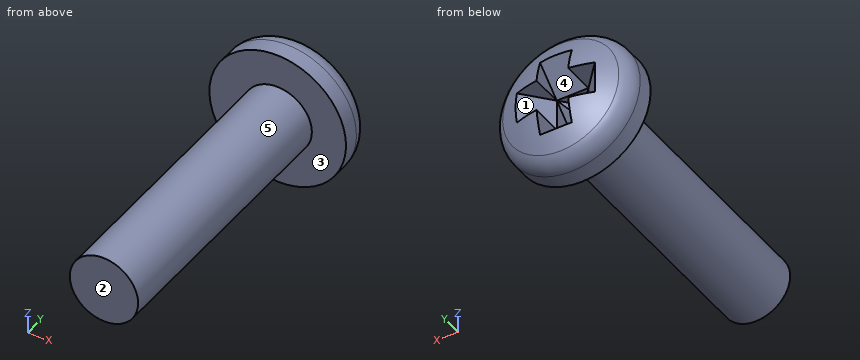
```python
from build123d import *

# Parameters (mm, degrees)
SKETCH2_W          = 1.5875
SKETCH2_H          = 12.7
CUT_EXTRUDE1_DEPTH = 0.736599362
CUT_EXTRUDE2_DEPTH = 0.736599362


with BuildPart() as part:
    # Sketch1 → Base-Revolve (revolve)
    with BuildSketch(Plane.XY, mode=Mode.PRIVATE) as base_revolve_sk:
        with BuildLine():
            Line((0, 0), (3.175, 0))
            Line((3.175, 0), (3.175, 0.762))
            ThreePointArc((3.175, 0.762), (3.047218091, 1.234139911), (2.698756382, 1.577387268))
            ThreePointArc((2.698756382, 1.577387268), (1.395118097, 2.105894374), (0, 2.286))
            Line((0, 2.286), (0, 0))
        make_face()
    revolve(base_revolve_sk.sketch.rotate(Axis((0, 0, 0), (0, 1, 0)), 90), axis=Axis((0, 0, 0), (0, 1, 0)))

    # Sketch2 → Boss-Revolve1 (revolve)
    with BuildSketch(Plane.XY):
        with Locations((0.79375, -6.35)):
            Rectangle(SKETCH2_W, SKETCH2_H)
    revolve(axis=Axis((0, 0, 0), (0, 1, 0)))

    # Sketch3 → Cut-Extrude1 (cut, symmetric)
    with BuildSketch(Plane.XY):
        Polygon((-4.038596502, 6.667494225), (4.038596502, 6.667494225), (4.038596502, 4.44499615), (0, -0.12699989), (-4.038596502, 4.44499615), align=None)
    extrude(amount=CUT_EXTRUDE1_DEPTH, both=True, mode=Mode.SUBTRACT)

    # Sketch4 → Cut-Extrude2 (cut, symmetric)
    with BuildSketch(Plane(origin=(0, 0, 0), x_dir=(0, 0, -1), z_dir=(1, 0, 0))):
        Polygon((-4.038596502, 6.667494225), (4.038596502, 6.667494225), (4.038596502, 4.44499615), (0, -0.12699989), (-4.038596502, 4.44499615), align=None)
    extrude(amount=CUT_EXTRUDE2_DEPTH, both=True, mode=Mode.SUBTRACT)


solid = part.part
```
For this review, take the finished solid that the model builds, in its own axes (mm). Face numbers are marked on the shaded views. A direction names the side the tool comes from. Coordinates: 2 decimals unless noted, no trailing zeros. Write each loop counter-clockwise with the first axis right and the second up, starting at its lowest first coordinate (ties: lowest second). Pieces come first, ordered by that corner, then holes.
(1) Tool access review of the marked faces 1 and 2: name each direction out of +Z, -Z, +X, -X, +Y, -Y from which nothing blocks a thin tool from reaching the whole face with its end or side.
(2) Wall thickness on probe 1 along Y at (x, z) = (-2, 1); probe 2 along Z at (x, y) = (-1.25, 1.75); probe 3 along Z at (x, y) = (0, -11.5): over which ranges is each line inside the solid? List them lowest first.
(3) For pin 1 Ø0.5 at (x, y) = (1.5, 1.5) entering from +Z; pin 2 Ø0.7 at (x, y) = (0.5, 0.5) entering from -Z; pin 3 Ø1.2 at (y, z) = (1, 1.5) entering from -X; pin 4 Ø1 at (x, z) = (0, -2) entering from -Y, all flat-tipped, find the tip position at first contact; note any pin that passes through.
(4) Add section A-A on y = -10.5. Give the boundary of the cut face in (x, z) (1 decimal).
(5) The part is to be moulded in two halves that separate along Z. For the marked faces 3, 4 and 5, say which applies: +Z half, -Z half, draft (parallel to the pull), parting line (faces both ways), or undercut.
Answer sheet:
1. face 1: +Y
1. face 2: +Z, -Z, +X, -X, -Y
2. probe 1: y = 0 to 1.81
2. probe 2: z = -2.01 to -0.74, 0.74 to 2.01
2. probe 3: z = -1.59 to 1.59
3. pin 1: stops at z = 2.69
3. pin 2: stops at z = -3.17
3. pin 3: stops at x = -3.03
3. pin 4: stops at y = -12.7
4. outline: circle Ø3.2 at (0, 0)
5. face 3: draft
5. face 4: undercut
5. face 5: parting line
